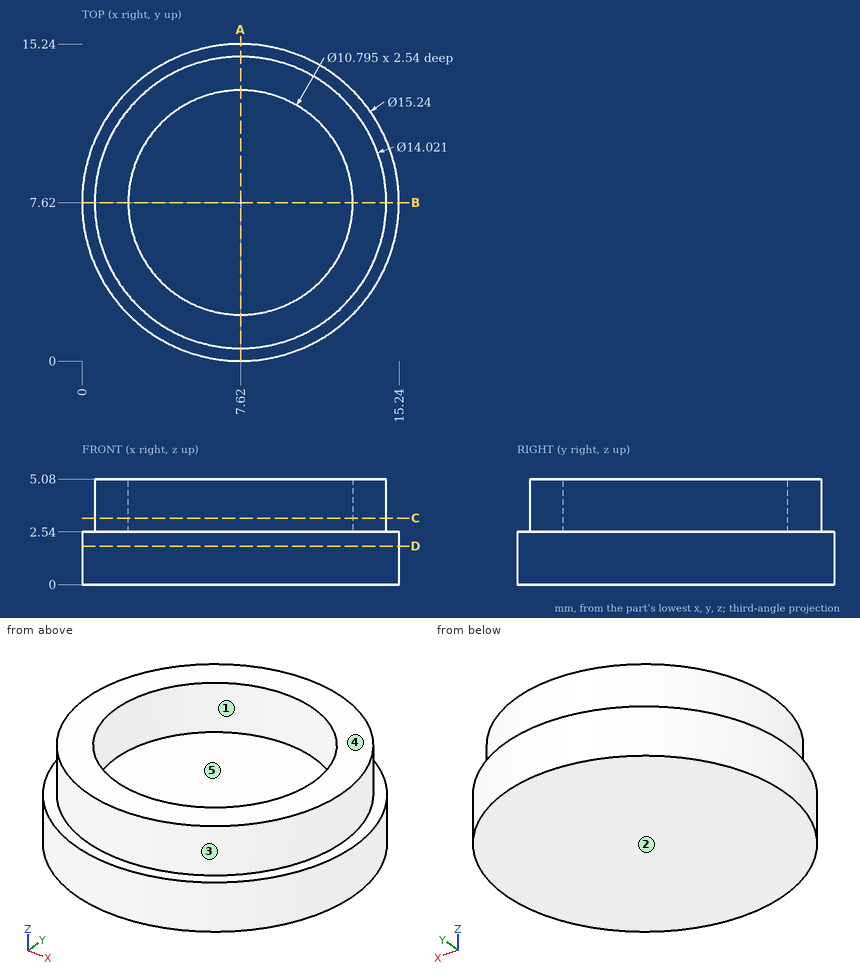
The drawing under review shows one solid part. Ordinate dimensions are in mm from its lowest x, y, z. A direction names the side the tool comes from. Round coordinates to 2 decimals unless told otherwise and drop trailing zeros. Order: outer loops, then holes, each group sorted by start corner. A loop starts at its lowest first (then second) coordinate and runs counter-clockwise, first axis right, second up. Notation, with made-up numbers: (-15, 22.5) -> (42, 22.5) arc R20 cw to (42, 38.5) -> close; hole circle Ø3 at (-33.5, 79). An arc over 180 degrees is marked (long way). Return JSON: item names as keys, results as strings.
1. The part is to be moulded in two halves that separate along X. For the marked faces 3, 4 and 5, say which applies: +X half, -X half, draft (parallel to the pull), parting line (faces both ways), or undercut.
Answer block:
{"face 3": "parting line", "face 4": "draft", "face 5": "undercut"}
2. Take a section at D-D (z = 1.85). Write out the cut boundary in (x, y), then the cut area to 3 significant figures.
Answer block:
{"outline": "circle Ø15.24 at (7.62, 7.62)", "area": "182 mm²"}
3. For the marked faces 1 and 2, list the 3-axis set-ups (+Z, -Z, +X, -X, +Y, -Y) from which the entire face can be reached by the end or side of a thin tool; tool diameter is ignored.
Answer block:
{"face 1": "+Z", "face 2": "-Z, +X, -X, +Y, -Y"}
4. Insertion check: P1, Ø7.5, axis at x = 7, y = 9, coming from the +Z side; P2, Ø1.5, axis at x = 4.5, z = 1.5, coming from the -Y side; P3, Ø4, axis at x = 8, y = 3.5, coming from the -Z side. Each pin has a flat end and moves straight along its axis. Give the tip position at first contact, or say it passes through.
Answer block:
{"P1": "stops at z = 2.54", "P2": "stops at y = 0.38", "P3": "stops at z = 0"}
5. For L1, parallel to Y at x = 7.62, z = 4; L2, parallel to Z at x = 3, y = 9.5; L3, parallel to Y at x = 7.5, z = 0.6, list the stretches that pass through material, from the lowest coordinate up. Write a range as [from, to].
Answer block:
{"L1": "y = [0.61, 2.22], [13.02, 14.63]", "L2": "z = [0, 2.54]", "L3": "y = [0, 15.24]"}
6. Take a section at A-A (x = 7.62). Write out the cut boundary in (y, z), then the cut area to 3 significant figures.
Answer block:
{"outline": "(0, 0) -> (15.24, 0) -> (15.24, 2.54) -> (14.63, 2.54) -> (14.63, 5.08) -> (13.02, 5.08) -> (13.02, 2.54) -> (2.22, 2.54) -> (2.22, 5.08) -> (0.61, 5.08) -> (0.61, 2.54) -> (0, 2.54) -> close", "area": "46.9 mm²"}
7. Take a section at C-C (z = 3.2). Write out the cut boundary in (x, y) (1 decimal).
Answer block:
{"outline": "circle Ø14 at (7.6, 7.6); hole circle Ø10.8 at (7.6, 7.6)"}
